Input: part model. Units: mm. Frame: model coordinates. Coordinates: 2 decimals unless noted, no trailing zeros. Write each loop counter-clockwise with the first axis right and the second up, starting at its lowest first coordinate (ties: lowest second). Pieces come first, ordered by that corner, then holes. Notation, with made-up numbers: (-31.75, 74.25) - (-4.75, 74.25) arc R31 ccw to (-4.75, 104.25) - close; hole circle Ø5 at (-16.75, 88.25). An arc over 180 degrees is marked (long way). Put each result on its own line as item: value. Start each with the question number.
1. Cut plane B-B, the plane x = 84. Return loops of the section in (y, z).
2. Cut plane A-A, the plane z = 0.6. Count the separate pieces of the cut face and the enclosed holes in it, and give its area (3 significant figures).
3. Line query: line 1 (Y direction, x = -90.5, z = 0.9). Output: solid intervals per line, ascending.
from build123d import *

# Parameters (mm, degrees)
SKETCH1_R           = 1.65
BOSS_EXTRUDE1_DEPTH = 1
SKETCH2_W           = 5
SKETCH2_H           = 0.1
CUT_EXTRUDE1_DEPTH  = 0.1


with BuildPart() as part:
    # Sketch1 → Boss-Extrude1 (new body)
    with BuildSketch(Plane.XY):
        Polygon((-140, 135), (-100, 135), (-100, 145), (-95, 145), (-95, 135), (95, 135), (95, 145), (100, 145), (100, 135), (140, 135), (140, -135), (-140, -135), align=None)
        with Locations((-133.5, 0)):
            Circle(SKETCH1_R, mode=Mode.SUBTRACT)
        with Locations((-133.5, 26.25)):
            Circle(SKETCH1_R, mode=Mode.SUBTRACT)
        with Locations((-133.5, 52.5)):
            Circle(SKETCH1_R, mode=Mode.SUBTRACT)
        with Locations((-133.5, 78.75)):
            Circle(SKETCH1_R, mode=Mode.SUBTRACT)
        with Locations((-133.5, 105)):
            Circle(SKETCH1_R, mode=Mode.SUBTRACT)
        with Locations((-133.5, -26.25)):
            Circle(SKETCH1_R, mode=Mode.SUBTRACT)
        with Locations((-133.5, -52.5)):
            Circle(SKETCH1_R, mode=Mode.SUBTRACT)
        with Locations((-133.5, -78.75)):
            Circle(SKETCH1_R, mode=Mode.SUBTRACT)
        with Locations((-133.5, -105)):
            Circle(SKETCH1_R, mode=Mode.SUBTRACT)
        with Locations(Location((133.5, -105, 0), (0, 0, 180))):
            Circle(SKETCH1_R, mode=Mode.SUBTRACT)
        with Locations(Location((133.5, -78.75, 0), (0, 0, 180))):
            Circle(SKETCH1_R, mode=Mode.SUBTRACT)
        with Locations(Location((133.5, -52.5, 0), (0, 0, 180))):
            Circle(SKETCH1_R, mode=Mode.SUBTRACT)
        with Locations(Location((133.5, -26.25, 0), (0, 0, 180))):
            Circle(SKETCH1_R, mode=Mode.SUBTRACT)
        with Locations(Location((133.5, 105, 0), (0, 0, 180))):
            Circle(SKETCH1_R, mode=Mode.SUBTRACT)
        with Locations(Location((133.5, 78.75, 0), (0, 0, 180))):
            Circle(SKETCH1_R, mode=Mode.SUBTRACT)
        with Locations(Location((133.5, 52.5, 0), (0, 0, 180))):
            Circle(SKETCH1_R, mode=Mode.SUBTRACT)
        with Locations(Location((133.5, 26.25, 0), (0, 0, 180))):
            Circle(SKETCH1_R, mode=Mode.SUBTRACT)
        with Locations(Location((133.5, 0, 0), (0, 0, 180))):
            Circle(SKETCH1_R, mode=Mode.SUBTRACT)
    extrude(amount=BOSS_EXTRUDE1_DEPTH)

    # Sketch2 → Cut-Extrude1 (cut)
    with BuildSketch(Plane.XY.offset(1)):
        with Locations((-97.5, 135.05)):
            Rectangle(SKETCH2_W, SKETCH2_H)
        with Locations((97.5, 135.05)):
            Rectangle(SKETCH2_W, SKETCH2_H)
    extrude(amount=-CUT_EXTRUDE1_DEPTH, mode=Mode.SUBTRACT)


solid = part.part
Report:
1. outline: (-135, 0) - (135, 0) - (135, 1) - (-135, 1) - close
2. separate pieces: 1
2. enclosed holes: 18
2. area: 75,500 mm^2
3. line 1: y = -135 to 135
